Autodesk Inventor part; units mm, degrees
ref_plane "YZ Plane" through (0, 0, 0) normal (1, 0, 0) x (0, 1, 0)
ref_plane "XZ Plane" through (0, 0, 0) normal (0, 1, 0) x (-1, 0, 0)
ref_plane "XY Plane" through (0, 0, 0) normal (0, 0, 1) x (1, 0, 0)
sketch "Sketch1" plane through (0, 0, 0) normal (1, 0, 0) x (0, 1, 0)
  line L0 (0, 0) -> (0, -292.1)
  arc A0 (0, 0) -> (0, -292.1) centre (0, -146.05) ccw
  dimension "d0" = 292.1
  dimension "d1" = 146.05
extrude "Extrusion1" add sketch "Sketch1" along normal blind 63.5
shell "Shell1" thickness 2.54 removed faces 1 at (42.3333, 0, -97.3667)
sketch "Sketch3" plane through (63.5, 0, 0) normal (1, 0, 0) x (0, 0, -1)
  line L0 (292.1, 0) -> (0, 0)
  line L1 (123.4186, 0) -> (168.6814, 0)
  line L2 (123.4186, 0) -> (123.4186, -144.4974)
  line L3 (168.6814, 0) -> (168.6814, -144.4974)
  arc A0 (2.54, 0) -> (289.56, 0) centre (146.05, 0) ccw
  arc A1 (123.4186, -141.5071) -> (168.6814, -141.7143) centre (146.663, -7.7251) ccw
  dimension "d9" = 45.2628
  dimension "d10" = 123.4186
extrude "Extrusion4" cut sketch "Sketch3" against normal blind 3810000 contours L3 A0 A1 L2 L0 | A1 A0
properties part number "GearHolster"
The listing builds one solid part. Answer for the finished solid, in the listing's coordinates (mm). A direction names the side the tool comes from. Coordinates: 2 decimals unless noted, no trailing zeros. Order: outer loops, then holes, each group sorted by start corner. A loop starts at its lowest first (then second) coordinate and runs counter-clockwise, first axis right, second up. Notation, with made-up numbers: M 63,15 L 84,15 A18 ccw 84,21 Z; hole C -40,38.5 d11. An arc over 180 degrees is marked long. Answer as a JSON object with one key per item and string values. Group by question number.
1. Flat-ended cylindrical pins translate along their axes: P1, Ø0.8, axis at x = 62, y = -100.5, coming from the -Z side; P2, Ø1.5, axis at x = 6.5, y = -84.5, coming from the +Z side; P3, Ø2, axis at x = 1, y = -68.5, coming from the -Z side. Find the tip coordinate at first contact, or state that the pin passes through.
2. Determine the mould class of faces 3 (the flat face through (62, 0, -43)), 4 (the cylindrical face through (31.306, -146.015, -149.262)), 5 (the flat face through (2.54, -56, -215)) for opening direction Z: released by +Z, released by -Z, zero draft, split by the parting line, or undercut.
3. Section C-C on z = -18 is taken. Write down the section's boundary in (x, y), then the cut area to 3 significant figures.
4. A tool of negligible diameter and unlimited length cuts with its end or side. For faces 1 (the cylindrical face through (31.34, -102.58, -45.69)), 2 (the flat face through (0, -58, -176)), from which of +Z, -Z, +X, -X, +Y, -Y can it reach the whole face along a straight path? Write none if from no direction.
5. Straight lines are drawn through the part: line 1 (X direction, y = -103.5, z = -186.5); line 2 (Y direction, x = 37, z = -146.5); line 3 (Z direction, x = 45, y = -55.5). For each, find the intervals that lie inside material, in ascending order.
6. Section D-D on y = -32.5 is taken. Write down the section's boundary in (x, z), then the cut area to 3 significant figures.
7. Section B-B on x = 48 is taken. Write down the section's boundary in (y, z) (3 decimals).
8. Section A-A on y = -117.5 is taken. Write down the section's boundary in (x, z), then the cut area to 3 significant figures.
Values follow:
{
 "1": {"P1": "z = -252.4", "P2": "z = -26.4", "P3": "z = -275.57"},
 "2": {"face 3": "zero draft", "face 4": "split by the parting line", "face 5": "undercut"},
 "3": {"outline": "M 0,-70.24 L 63.5,-70.24 L 63.5,0 L 60.96,0 L 60.96,-64.79 L 2.54,-64.79 L 2.54,0 L 0,0 Z", "area": "675 mm2"},
 "4": {"face 1": "+Y", "face 2": "+Z, -Z, -X, +Y, -Y"},
 "5": {"line 1": "0 to 2.54, 60.96 to 63.5", "line 2": "-146.05 to -143.51", "line 3": "-281.14 to -278.39, -13.71 to -10.96"},
 "6": {"outline": "M 0,-288.44 L 63.5,-288.44 L 63.5,-168.68 L 60.96,-168.68 L 60.96,-285.83 L 2.54,-285.83 L 2.54,-168.68 L 0,-168.68 Z; M 0,-123.42 L 2.54,-123.42 L 2.54,-6.27 L 60.96,-6.27 L 60.96,-123.42 L 63.5,-123.42 L 63.5,-3.66 L 0,-3.66 Z", "area": "1,520 mm2"},
 "7": {"outline": "M -143.51,-146.041 A143.51 cw 0,-2.54 L 0,0 A146.05 ccw 0,-292.1 L 0,-289.56 A143.51 cw -141.714,-168.681 A135.785 cw Z"},
 "8": {"outline": "M 0,-232.79 L 63.5,-232.79 L 63.5,-168.68 L 60.96,-168.68 L 60.96,-228.44 L 2.54,-228.44 L 2.54,-168.68 L 0,-168.68 Z; M 0,-123.42 L 2.54,-123.42 L 2.54,-63.66 L 60.96,-63.66 L 60.96,-123.42 L 63.5,-123.42 L 63.5,-59.31 L 0,-59.31 Z", "area": "1,160 mm2"}
}
